Can you work these out from the drawing? Everything is in mm from the part's minimum corner. A direction names the side the tool comes from. Round coordinates to 2 decimals unless told otherwise and drop trailing zeros. Order: outer loops, then holes, each group sorted by start corner. A loop starts at its lowest first (then second) coordinate and runs counter-clockwise, first axis right, second up. Notation, with made-up numbers: (-34.75, -10) -> (13.25, -10) arc R21 cw to (13.25, 5) -> close; hole circle Ø11 at (83.25, 4.5). An arc over 180 degrees is marked (long way). One line per item, written item: value.
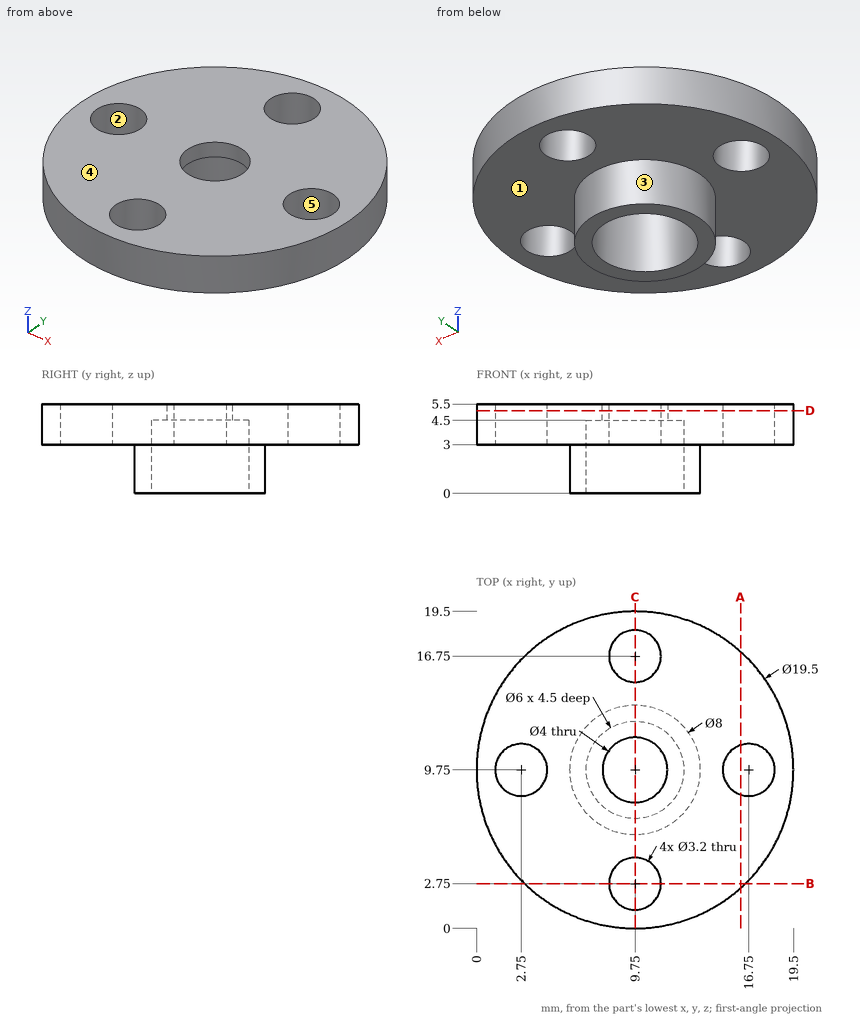
Q1. I want a section at A-A on x = 16.25. List the corners of the cut face in (y, z) for me, plus the area to 3 significant figures.
Answers below:
outline: (2.48, 3) -> (8.23, 3) -> (8.23, 5.5) -> (2.48, 5.5) -> close; (11.27, 3) -> (17.02, 3) -> (17.02, 5.5) -> (11.27, 5.5) -> close
area: 28.7 mm^2
Q2. We'd pull the mould along Y, two halves only. Please class the marked faces 3, 4 and 5: released by +Y, released by -Y, zero draft, split by the parting line, or undercut.
Answers below:
face 3: split by the parting line
face 4: zero draft
face 5: undercut
Q3. On a 3-axis mill with a long thin cutter (end or side, diameter ignored), from which of +Z, -Z, +X, -X, +Y, -Y can I reach the whole of each face in a straight line? I mean the marked faces 1 and 2. Say none if no direction works.
Answers below:
face 1: -Z
face 2: +Z, -Z
Q4. Please list where these lines run through material, in increasing order: line 1 along Y through (x, z) = (9.75, 3.6); line 2 along X through (y, z) = (9.25, 4.85); line 3 along Z through (x, y) = (2.5, 7.5).
Answers below:
line 1: 0 to 1.15, 4.35 to 6.75, 12.75 to 15.15, 18.35 to 19.5
line 2: 0.01 to 1.23, 4.27 to 7.81, 11.69 to 15.23, 18.27 to 19.49
line 3: 3 to 5.5
Q5. I want a section at D-D on z = 5.1. List the corners of the cut face in (x, y) for me.
Answers below:
outline: circle Ø19.5 at (9.75, 9.75); hole circle Ø3.2 at (2.75, 9.75); hole circle Ø4 at (9.75, 9.75); hole circle Ø3.2 at (9.75, 2.75); hole circle Ø3.2 at (9.75, 16.75); hole circle Ø3.2 at (16.75, 9.75)
Q6. I want a section at C-C on x = 9.75. List the corners of the cut face in (y, z) for me, plus the area to 4 significant figures.
Answers below:
outline: (0, 3) -> (1.15, 3) -> (1.15, 5.5) -> (0, 5.5) -> close; (4.35, 3) -> (5.75, 3) -> (5.75, 0) -> (6.75, 0) -> (6.75, 4.5) -> (7.75, 4.5) -> (7.75, 5.5) -> (4.35, 5.5) -> close; (11.75, 4.5) -> (12.75, 4.5) -> (12.75, 0) -> (13.75, 0) -> (13.75, 3) -> (15.15, 3) -> (15.15, 5.5) -> (11.75, 5.5) -> close; (18.35, 3) -> (19.5, 3) -> (19.5, 5.5) -> (18.35, 5.5) -> close
area: 25.75 mm^2
Q7. Will these pins go through, and if not, where does the flat tip stop? pin 1 Ø1.9 at (x, y) = (9.75, 2.75) entering from -Z; pin 2 Ø3 at (x, y) = (4, 13.5) entering from -Z; pin 3 Ø1 at (y, z) = (17, 3.5) entering from -X; pin 4 Ø2 at (y, z) = (7, 2.5) entering from +X.
Answers below:
pin 1: through
pin 2: z = 3
pin 3: x = 2.71
pin 4: x = 19.32
Q8. I want a section at B-B on y = 2.75. List the corners of the cut face in (x, z) for me, plus the area to 3 significant figures.
Answers below:
outline: (2.96, 3) -> (8.15, 3) -> (8.15, 5.5) -> (2.96, 5.5) -> close; (11.35, 3) -> (16.54, 3) -> (16.54, 5.5) -> (11.35, 5.5) -> close
area: 25.9 mm^2
